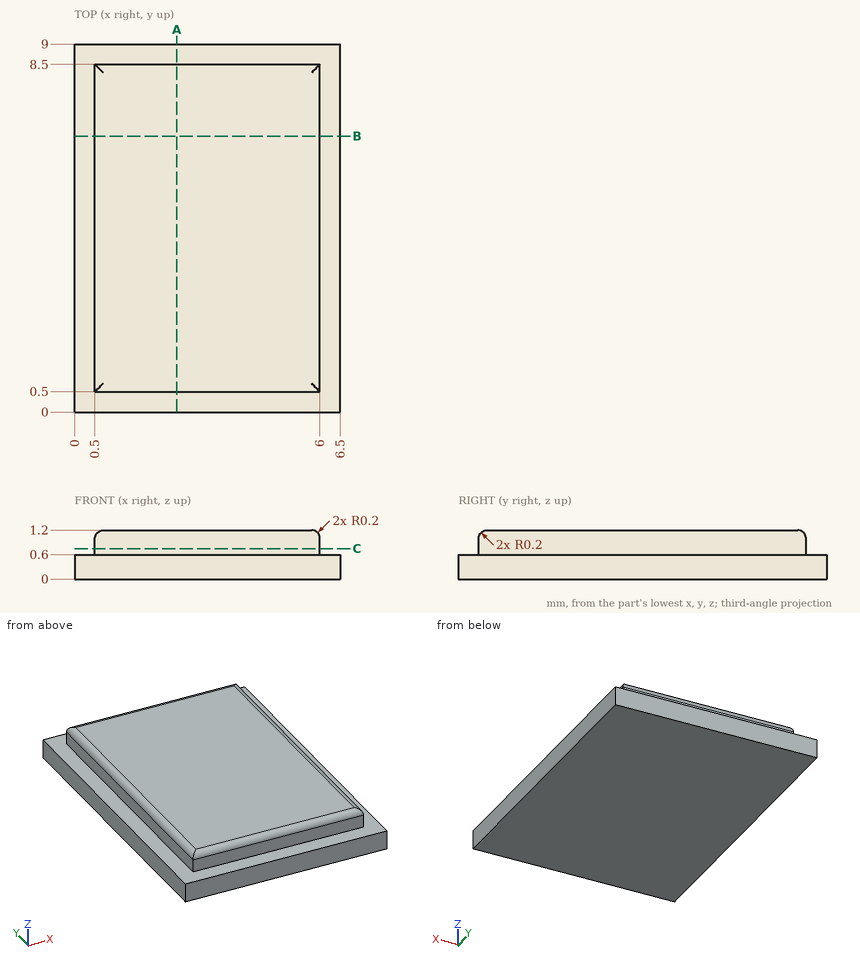
Input: dimensioned drawing with shaded views. Units: mm. Origin: part minimum x, y, z. Round coordinates to 2 decimals unless told otherwise and drop trailing zeros. Order: outer loops, then holes, each group sorted by start corner. A loop starts at its lowest first (then second) coordinate and runs counter-clockwise, first axis right, second up.
Q1. Material intervals for probe 1 along X at (y, z) = (0.75, 0.7); probe 2 along Y at (x, z) = (1.25, 0.9); probe 3 along Z at (x, y) = (6.25, 5.5), sorted ascending.
Result sheet:
probe 1: x = 0.5 to 6
probe 2: y = 0.5 to 8.5
probe 3: z = 0 to 0.6
Q2. Section B-B, the plane y = 6.75. Output: boundary loops of the cut face in (x, z).
Result sheet:
outline: (0, 0) - (6.5, 0) - (6.5, 0.6) - (6, 0.6) - (6, 1) arc R0.2 ccw to (5.8, 1.2) - (0.7, 1.2) arc R0.2 ccw to (0.5, 1) - (0.5, 0.6) - (0, 0.6) - close
Q3. Section C-C, the plane z = 0.75. Output: boundary loops of the cut face in (x, y), and give its area (3 significant figures).
Result sheet:
outline: (0.5, 0.5) - (6, 0.5) - (6, 8.5) - (0.5, 8.5) - close
area: 44.0 mm2
Q4. Section A-A, the plane x = 2.5. Output: boundary loops of the cut face in (y, z).
Result sheet:
outline: (0, 0) - (9, 0) - (9, 0.6) - (8.5, 0.6) - (8.5, 1) arc R0.2 ccw to (8.3, 1.2) - (0.7, 1.2) arc R0.2 ccw to (0.5, 1) - (0.5, 0.6) - (0, 0.6) - close
